from build123d import *

# Parameters (mm, degrees)
BOSS_EXTRUDE1_DEPTH       = 30
CHAMFER1_SIZE             = 10
FILLET1_R                 = 6
F_5_0MM_DOWEL_HOLE1_D     = 5
F_5_0MM_DOWEL_HOLE1_DEPTH = 12
F_5_0MM_DOWEL_HOLE1_TIP   = 1.502151548
CHAMFER2_SIZE             = 0.4


with BuildPart() as part:
    # Sketch1 → Boss-Extrude1 (new body)
    with BuildSketch(Plane(origin=(0, 0, 0), x_dir=(1, 0, 0), z_dir=(0, 1, 0))):
        Polygon((-45, 30), (-45, -12), (45, -12), (45, 30), (27.2, 30), (27.2, 0), (-27.2, 0), (-27.2, 30), align=None)
    extrude(amount=BOSS_EXTRUDE1_DEPTH)

    # Chamfer1
    chamfer1_edges = [part.edges().sort_by_distance(p)[0] for p in [
        (45, 15, 12),
        (-45, 15, 12),
    ]]
    chamfer(chamfer1_edges, length=CHAMFER1_SIZE)

    # Fillet1
    fillet1_edges = [part.edges().sort_by_distance(p)[0] for p in [
        (-45, 0, -14),
        (45, 0, -14),
        (45, 30, -14),
        (-45, 30, -14),
    ]]
    fillet(fillet1_edges, radius=FILLET1_R)

    # Ø5.0mm Dowel Hole1
    with Locations(Plane(origin=(0, 0, -30), x_dir=(-1, 0, 0), z_dir=(0, 0, -1))):
        with Locations((-36.1, 7.5), (36.1, 22.5), (36.1, 7.5), (-36.1, 22.5)):
            Hole(F_5_0MM_DOWEL_HOLE1_D / 2, depth=F_5_0MM_DOWEL_HOLE1_DEPTH)
            with Locations((0, 0, -(F_5_0MM_DOWEL_HOLE1_DEPTH + F_5_0MM_DOWEL_HOLE1_TIP / 2))):  # 118° drill point
                Cone(0, F_5_0MM_DOWEL_HOLE1_D / 2, F_5_0MM_DOWEL_HOLE1_TIP, mode=Mode.SUBTRACT)

    # Chamfer2
    chamfer2_edges = [part.edges().sort_by_distance(p)[0] for p in [
        (-33.1, 0, -30),
        (-27.2, 15, -30),
        (27.2, 15, -30),
        (27.2, 30, -15),
        (0, 30, 0),
        (-27.2, 30, -15),
        (33.1, 30, -30),
        (-45, 15, -30),
        (-43.242640687, 1.757359313, -30),
        (-43.242640687, 28.242640687, -30),
        (33.1, 0, -30),
        (45, 15, -30),
        (43.242640687, 1.757359313, -30),
        (-33.1, 30, -30),
        (43.242640687, 28.242640687, -30),
        (33.6, 7.5, -30),
        (33.6, 22.5, -30),
        (-38.6, 7.5, -30),
        (-38.6, 22.5, -30),
        (-27.2, 0, -15),
        (0, 0, 0),
        (27.2, 0, -15),
    ]]
    chamfer(chamfer2_edges, length=CHAMFER2_SIZE)


solid = part.part
The listing builds one solid part. Answer for the finished solid, in the listing's coordinates (mm). A direction names the side the tool comes from. Coordinates: 2 decimals unless noted, no trailing zeros. Order: outer loops, then holes, each group sorted by start corner. A loop starts at its lowest first (then second) coordinate and runs counter-clockwise, first axis right, second up. Notation, with made-up numbers: (77, 86) -> (117, 86) arc R25 ccw to (117, 101) -> close; hole circle Ø11 at (20.25, 89). An arc over 180 degrees is marked (long way). Answer in a Markdown table with one row per item. Add a question column.
Item 1: Determine the mould class of faces 4 (the face through (43.196, 28.289, -11.063)), 5 (the face through (-36.33, 7.87, -16.76)), 6 (the face through (-36, 15, -30)) for opening direction X: +X half, -X half, draft (parallel to the pull), parting line (faces both ways), or undercut.
Item 2: Find section C-C (y = 16.5). Write down the section's boundary in (x, z), then the cut area to 3 significant figures.
Item 3: Find section B-B (z = -4.5). Write down the section's boundary in (x, y).
Item 4: Find the intervals of material crossed by L1, parallel to X at y = 7.5, z = -22.25; L2, parallel to Y at x = -36.1, z = -25.5; L3, parallel to X at y = 22, z = -20, in increasing order. Write a range as from..to.
Item 5: Find section D-D (x = 10). Write down the section's boundary in (y, z).
Item 6: Each of these flat-tipped pins is pushed along its axis until it touches: P1, Ø4, axis at x = 36.1, y = 22.5, coming from the -Z side; P2, Ø1, axis at x = -13, y = 19.5, coming from the -Z side. Where does it stop, or does it pass through?
Item 7: Which of the six approach directions +Z, -Z, +X, -X, +Y, -Y give full straight-line access (tool end or side, diameter ignored) to faces 1 (the face through (-40, 15, 7)), 2 (the face through (-27.2, 15, -15)), 3 (the face through (-33.79, 6.54, -23.72))?
Item 8: Find section A-A (z = -20.5). Write down the section's boundary in (x, y).
Result set:
| question | item | result |
|---|---|---|
| 1 | face 4 | +X half |
| 1 | face 5 | undercut |
| 1 | face 6 | draft |
| 2 | outline | (-45, -29.6) -> (-44.6, -30) -> (-27.6, -30) -> (-27.2, -29.6) -> (-27.2, 0) -> (27.2, 0) -> (27.2, -29.6) -> (27.6, -30) -> (44.6, -30) -> (45, -29.6) -> (45, 2) -> (35, 12) -> (-35, 12) -> (-45, 2) -> close |
| 2 | area | 2,050 mm² |
| 3 | outline | (-45, 6) arc R6 ccw to (-39, 0) -> (-27.6, 0) -> (-27.2, 0.4) -> (-27.2, 29.6) -> (-27.6, 30) -> (-39, 30) arc R6 ccw to (-45, 24) -> close; (27.2, 0.4) -> (27.6, 0) -> (39, 0) arc R6 ccw to (45, 6) -> (45, 24) arc R6 ccw to (39, 30) -> (27.6, 30) -> (27.2, 29.6) -> close |
| 4 | L1 | x = -45..-38.6, -33.6..-27.2, 27.2..33.6, 38.6..45 |
| 4 | L2 | y = 0..5, 10..20, 25..30 |
| 4 | L3 | x = -45..-38.55, -33.65..-27.2, 27.2..33.65, 38.55..45 |
| 5 | outline | (0, 0.4) -> (0.4, 0) -> (29.6, 0) -> (30, 0.4) -> (30, 12) -> (0, 12) -> close |
| 6 | P1 | stops at z = -17.7 |
| 6 | P2 | stops at z = 0 |
| 7 | face 1 | +Z, -X, +Y, -Y |
| 7 | face 2 | -Z, +Y, -Y |
| 7 | face 3 | -Z |
| 8 | outline | (-45, 6) arc R6 ccw to (-39, 0) -> (-27.6, 0) -> (-27.2, 0.4) -> (-27.2, 29.6) -> (-27.6, 30) -> (-39, 30) arc R6 ccw to (-45, 24) -> close; (27.2, 0.4) -> (27.6, 0) -> (39, 0) arc R6 ccw to (45, 6) -> (45, 24) arc R6 ccw to (39, 30) -> (27.6, 30) -> (27.2, 29.6) -> close; hole circle Ø5 at (-36.1, 7.5); hole circle Ø5 at (-36.1, 22.5); hole circle Ø5 at (36.1, 7.5); hole circle Ø5 at (36.1, 22.5) |
